Input: part model. Units: mm. Frame: model coordinates. A direction names the side the tool comes from. Give positions to 0.01 mm unless a question says otherwise; leave off trailing zeros. Order: outer loops, then holes, each group sorted by start corner. A loop starts at its lowest first (then second) coordinate and runs counter-clockwise, first axis right, second up. Notation, with made-up numbers: (29, 14) -> (56, 14) arc R15 cw to (56, 31) -> close; hole circle Ø11 at (36.5, 47). An arc over 180 degrees is marked (long way). Use a Markdown table: item, result. Add a question column.
from build123d import *

# Parameters (mm, degrees)
F0_W     = 2
F0_H     = 7
F0_W_2   = 5
F0_R     = 0.98
F1_DEPTH = 2
F2_DEPTH = 8
F3_W     = 3.5
F3_H     = 1.5
F4_DEPTH = 25
F5_R     = 0.5


with BuildPart() as f1:
    # F0 (on Top) → F1 (new body)
    with BuildSketch(Plane.XY):
        with Locations((-3.5, 0)):
            Rectangle(F0_W, F0_H)
        Rectangle(F0_W_2, F0_H)
        Circle(F0_R, mode=Mode.SUBTRACT)
        with Locations((3.5, 0)):
            Rectangle(F0_W, F0_H)
    extrude(amount=-F1_DEPTH)

    # F0 (on Top) → F2 (join)
    with BuildSketch(Plane.XY):
        with Locations((-3.5, 0)):
            Rectangle(F0_W, F0_H)
        with Locations((3.5, 0)):
            Rectangle(F0_W, F0_H)
    extrude(amount=F2_DEPTH)

    # F3 (on face) → F4 (cut)
    with BuildSketch(Plane(origin=(-4.5, 0, 0), x_dir=(0, -1, 0), z_dir=(-1, 0, 0))):
        with Locations((0, 5.75)):
            Rectangle(F3_W, F3_H)
    extrude(amount=-F4_DEPTH, mode=Mode.SUBTRACT)

    # F5
    f5_edges = [f1.edges().sort_by_distance(p)[0] for p in [
        (-2.5, -3.5, 4),
        (-4.5, 0, 8),
        (-2.5, 0, 8),
        (2.5, 0, 8),
        (4.5, 0, 8),
        (2.5, -3.5, 4),
        (4.5, -3.5, 3),
        (-4.5, -3.5, 3),
        (-4.5, 3.5, 3),
        (2.5, 3.5, 4),
        (4.5, 3.5, 3),
        (-2.5, 3.5, 4),
        (0, -3.5, 0),
        (0, 3.5, 0),
    ]]
    fillet(f5_edges, radius=F5_R)


solid = f1.part
Q1. Draft query along X for faces 1 (the cylindrical face through (-0.212, -0.957, -0.986)), 2 (the flat face through (4.5, 0, 3)), 3 (the flat face through (0, -3.5, -1)), 4 (the flat face through (2.5, 0, 4)). Return one class per face: +X half, -X half, draft (parallel to the pull), parting line (faces both ways), or undercut.
Q2. First-contact query: pin 1 (1.5 mm diameter, centred on x = -1, y = 0, fed in from +Z); pin 2 (4 mm diameter, centred on x = 1.5, z = 1.5, fed in from +Y). Flat tips, straight axial feed; report the tip coordinate or a pass-through.
Q3. Section query A-A (x = 0). Return loops of the section in (y, z).
Q4. Section query D-D (y = -2.75). Return loops of the section in (x, z).
Q5. Ray query, line 1 (Z direction, x = -3.5, y = 0.5); line 2 (X direction, y = 1, z = 0.25); line 3 (Y direction, x = 0, z = -1.25). Return the intervals inside material, ascending.
Q6. Section query C-C (y = 0). Return loops of the section in (x, z), plus the area to 3 significant figures.
Q7. Section query B-B (z = 2.5). Return loops of the section in (x, y), plus the area to 3 significant figures.
Q8. Access query for faces 5 (the flat face through (-1, 1, -2)), 6 (the flat face through (-2.5, 0, 4)), 7 (the flat face through (-4, 0, 5)). Directions: +Z, -Z, +X, -X, +Y, -Y. A direction counts if a zero-diameter tool reaches every point of the face in a straight line with its end or side. Return the directions, or none.
Solution:
| question | item | result |
|---|---|---|
| 1 | face 1 | undercut |
| 1 | face 2 | +X half |
| 1 | face 3 | draft |
| 1 | face 4 | undercut |
| 2 | pin 1 | stops at z = 0 |
| 2 | pin 2 | stops at y = 3.5 |
| 3 | outline | (-3.5, -2) -> (-0.98, -2) -> (-0.98, 0) -> (-3, 0) arc R0.5 ccw to (-3.5, -0.5) -> close; (0.98, -2) -> (3.5, -2) -> (3.5, -0.5) arc R0.5 ccw to (3, 0) -> (0.98, 0) -> close |
| 4 | outline | (-4.5, -2) -> (4.5, -2) -> (4.5, 7.5) arc R0.5 ccw to (4, 8) -> (3, 8) arc R0.5 ccw to (2.5, 7.5) -> (2.5, 0) -> (-2.5, 0) -> (-2.5, 7.5) arc R0.5 ccw to (-3, 8) -> (-4, 8) arc R0.5 ccw to (-4.5, 7.5) -> close |
| 5 | line 1 | z = -2 to 5, 6.5 to 8 |
| 5 | line 2 | x = -4.5 to -2.5, 2.5 to 4.5 |
| 5 | line 3 | y = -3.5 to -0.98, 0.98 to 3.5 |
| 6 | outline | (-4.5, -2) -> (-0.98, -2) -> (-0.98, 0) -> (-2.5, 0) -> (-2.5, 5) -> (-4.5, 5) -> close; (-4.5, 6.5) -> (-2.5, 6.5) -> (-2.5, 7.5) arc R0.5 ccw to (-3, 8) -> (-4, 8) arc R0.5 ccw to (-4.5, 7.5) -> close; (0.98, -2) -> (4.5, -2) -> (4.5, 5) -> (2.5, 5) -> (2.5, 0) -> (0.98, 0) -> close; (2.5, 6.5) -> (4.5, 6.5) -> (4.5, 7.5) arc R0.5 ccw to (4, 8) -> (3, 8) arc R0.5 ccw to (2.5, 7.5) -> close |
| 6 | area | 39.9 mm² |
| 7 | outline | (-4.5, -3) arc R0.5 ccw to (-4, -3.5) -> (-3, -3.5) arc R0.5 ccw to (-2.5, -3) -> (-2.5, 3) arc R0.5 ccw to (-3, 3.5) -> (-4, 3.5) arc R0.5 ccw to (-4.5, 3) -> close; (2.5, -3) arc R0.5 ccw to (3, -3.5) -> (4, -3.5) arc R0.5 ccw to (4.5, -3) -> (4.5, 3) arc R0.5 ccw to (4, 3.5) -> (3, 3.5) arc R0.5 ccw to (2.5, 3) -> close |
| 7 | area | 27.6 mm² |
| 8 | face 5 | -Z, +X, -X, +Y, -Y |
| 8 | face 6 | +Z, +Y, -Y |
| 8 | face 7 | +X, -X |
